```python
from build123d import *

# Parameters (mm, degrees)
SKETCH1_R           = 2.4892
BOSS_EXTRUDE1_DEPTH = 3.175
FILLET1_R           = 4.7625


with BuildPart() as part:
    # Sketch1 → Boss-Extrude1 (new body)
    with BuildSketch(Plane.XY):
        Polygon((28.575, -2.54), (61.976, -2.54), (61.976, -63.5), (45.72, -63.5), (45.72, -24.13), (28.575, -24.13), align=None)
        with Locations((53.975, -27.94)):
            Circle(SKETCH1_R, mode=Mode.SUBTRACT)
        with Locations((53.975, -40.64)):
            Circle(SKETCH1_R, mode=Mode.SUBTRACT)
        with Locations((53.975, -53.34)):
            Circle(SKETCH1_R, mode=Mode.SUBTRACT)
        with Locations((34.925, -15.24)):
            Circle(SKETCH1_R, mode=Mode.SUBTRACT)
    extrude(amount=BOSS_EXTRUDE1_DEPTH)

    # Fillet1
    fillet1_edges = [part.edges().sort_by_distance(p)[0] for p in [
        (61.976, -63.5, 1.5875),
        (45.72, -63.5, 1.5875),
        (45.72, -24.13, 1.5875),
        (28.575, -24.13, 1.5875),
        (28.575, -2.54, 1.5875),
        (61.976, -2.54, 1.5875),
    ]]
    fillet(fillet1_edges, radius=FILLET1_R)


solid = part.part
```
Design review of the part built by this model. Coordinates are the model's own, in mm. A direction names the side the tool comes from. Coordinates: 2 decimals unless noted, no trailing zeros. Order: outer loops, then holes, each group sorted by start corner. A loop starts at its lowest first (then second) coordinate and runs counter-clockwise, first axis right, second up. Notation, with made-up numbers: (11.5, 23.25) -> (24.5, 23.25) arc R7 cw to (24.5, 30.25) -> close; hole circle Ø7 at (70.25, 28). An arc over 180 degrees is marked (long way). One line per item, written item: value. Start each with the question number.
Q1. Take a section at D-D, the plane y = -53.34. State the section outline as (x, z) points (3 decimals).
Q2. For probe 1 along Y at (x, z) = (55.5, 1.25); probe 2 along X at (y, z) = (-37, 2.75); probe 3 along Y at (x, z) = (54.5, 1.8), list the stretches that pass through material, from the lowest coordinate up.
Q3. Insertion check: pin 1 Ø1 at (x, z) = (38.5, 1) entering from -Y; pin 2 Ø1 at (y, z) = (-45.5, 1.5) entering from -X. Each pin has a flat end and moves straight along its axis. Give the tip position at first contact, or say it passes through.
Q4. Take a section at C-C, the plane x = 53.5. State the section outline as (y, z) points (3 decimals), then the cut area to 3 significant figures.
Q5. Take a section at B-B, the plane z = 1.65. State the section outline as (x, y) points (1 decimal), then the cut area to 3 significant figures.
Q6. Mouldability with a two-part tool opening along X and no side actions: class faces 3 (the cylindrical face through (53.651, -50.872, 1.565)), 4 (the flat face through (45, -2.54, 2)), 5 (the flat face through (45.72, -44, 2)) as pulls with the +X half, pulls with the -X half, needs draft (parallel to the pull), parting line crosses it, or undercut.
Q7. Tool access review of faces 1 (the flat face through (37, -24.13, 2)), 2 (the cylindrical face through (53.651, -38.172, 1.565)): name each direction out of +Z, -Z, +X, -X, +Y, -Y from which nothing blocks a thin tool from reaching the whole face with its end or side.
Q8. Take a section at A-A, the plane y = -15.24. State the section outline as (x, z) points (3 decimals).
Values follow:
1. outline: (45.72, 0) -> (51.486, 0) -> (51.486, 3.175) -> (45.72, 3.175) -> close; (56.464, 0) -> (61.976, 0) -> (61.976, 3.175) -> (56.464, 3.175) -> close
2. probe 1: y = -63.5 to -55.31, -51.37 to -42.61, -38.67 to -29.91, -25.97 to -2.54
2. probe 2: x = 45.72 to 61.98
2. probe 3: y = -63.5 to -55.77, -50.91 to -43.07, -38.21 to -30.37, -25.51 to -2.54
3. pin 1: stops at y = -24.13
3. pin 2: stops at x = 45.72
4. outline: (-63.5, 0) -> (-55.783, 0) -> (-55.783, 3.175) -> (-63.5, 3.175) -> close; (-50.897, 0) -> (-43.083, 0) -> (-43.083, 3.175) -> (-50.897, 3.175) -> close; (-38.197, 0) -> (-30.383, 0) -> (-30.383, 3.175) -> (-38.197, 3.175) -> close; (-25.497, 0) -> (-2.54, 0) -> (-2.54, 3.175) -> (-25.497, 3.175) -> close
4. area: 147 mm2
5. outline: (28.6, -19.4) arc R4.8 ccw to (33.3, -24.1) -> (41, -24.1) arc R4.8 cw to (45.7, -28.9) -> (45.7, -58.7) arc R4.8 ccw to (50.5, -63.5) -> (57.2, -63.5) arc R4.8 ccw to (62, -58.7) -> (62, -7.3) arc R4.8 ccw to (57.2, -2.5) -> (33.3, -2.5) arc R4.8 ccw to (28.6, -7.3) -> close; hole circle Ø5 at (34.9, -15.2); hole circle Ø5 at (54, -53.3); hole circle Ø5 at (54, -40.6); hole circle Ø5 at (54, -27.9)
5. area: 1,260 mm2
6. face 3: undercut
6. face 4: needs draft
6. face 5: pulls with the -X half
7. face 1: +Z, -Z, -X, -Y
7. face 2: +Z, -Z
8. outline: (28.575, 0) -> (32.436, 0) -> (32.436, 3.175) -> (28.575, 3.175) -> close; (37.414, 0) -> (61.976, 0) -> (61.976, 3.175) -> (37.414, 3.175) -> close
